from build123d import *

# Parameters (mm, degrees)
SKETCH2_W                                         = 184.171135827
SKETCH2_H                                         = 127
BOSS_EXTRUDE1_DEPTH                               = 4.7625
CSK_FOR_6_FLAT_HEAD_MACHINE_SCREW_100_D           = 4.3053
CSK_FOR_6_FLAT_HEAD_MACHINE_SCREW_100_CSINK_D     = 7.0866
CSK_FOR_6_FLAT_HEAD_MACHINE_SCREW_100_CSINK_ANGLE = 100
CUT_EXTRUDE1_DEPTH                                = 2440.147405433
F_2_CLEARANCE_HOLE1_D                             = 2.7051
CUT_EXTRUDE2_DEPTH                                = 4.7625
FILLET1_R                                         = 25.4
SKETCH10_W                                        = 30.7975
SKETCH10_H                                        = 54.356
CUT_EXTRUDE3_DEPTH                                = 2440.147405433
FILLET2_R                                         = 6.35
CUT_EXTRUDE4_DEPTH                                = 2440.147405433
FILLET3_R                                         = 12.7


with BuildPart() as part:
    # Sketch2 → Boss-Extrude1 (new body)
    with BuildSketch(Plane(origin=(-1e-09, -851.606445574, 6059.494718221), x_dir=(-1, 0, 0), z_dir=(1.0892556339675399e-13, 0.13917310096006327, -0.9902680687415707))):
        with Locations((-199.574242123, -2357.490725166)):
            Rectangle(SKETCH2_W, SKETCH2_H)
    extrude(amount=BOSS_EXTRUDE1_DEPTH)

    # CSK for #6 Flat Head Machine Screw (100)1 (through all)
    with Locations(Plane(origin=(-1e-09, -850.94363368, 6054.778566544), x_dir=(-1, 0, 0), z_dir=(1.0707755897952407e-13, 0.13917310096005847, -0.9902680687415714))):
        with Locations((-115.42617421, -2301.928225166), (-229.72617421, -2301.928225166), (-283.722310037, -2413.053225166)):
            CounterSinkHole(CSK_FOR_6_FLAT_HEAD_MACHINE_SCREW_100_D / 2, CSK_FOR_6_FLAT_HEAD_MACHINE_SCREW_100_CSINK_D / 2, counter_sink_angle=CSK_FOR_6_FLAT_HEAD_MACHINE_SCREW_100_CSINK_ANGLE)

    # Sketch5 → Cut-Extrude1 (cut, through all)
    with BuildSketch(Plane(origin=(-1e-09, -850.94363368, 6054.778566544), x_dir=(-1, 0, 0), z_dir=(1.0707755897952407e-13, 0.13917310096005847, -0.9902680687415714))):
        with BuildLine():
            Line((-195.975000021, -2361.610724808), (-195.975000021, -2336.210724808))
            ThreePointArc((-195.975000021, -2336.210724808), (-183.275000021, -2323.510724808), (-170.575000021, -2336.210724808))
            Line((-170.575000021, -2336.210724808), (-170.575000021, -2361.610724808))
            ThreePointArc((-170.575000021, -2361.610724808), (-183.275000021, -2374.310724808), (-195.975000021, -2361.610724808))
        make_face()
    extrude(amount=-CUT_EXTRUDE1_DEPTH, mode=Mode.SUBTRACT)

    # #2 Clearance Hole1 (through all)
    with Locations(Plane(origin=(-1e-09, -850.94363368, 6054.778566544), x_dir=(-1, 0, 0), z_dir=(1.0707755897952407e-13, 0.13917310096005847, -0.9902680687415714))):
        with Locations((-135.015000021, -2391.392725166), (-160.415000021, -2391.392725166), (-160.415000021, -2330.686725166), (-135.015000021, -2330.686725166), (-204.864100021, -2328.675325166), (-204.864100021, -2403.605325166), (-253.124100021, -2409.955325166), (-253.124100021, -2327.405325166)):
            Hole(F_2_CLEARANCE_HOLE1_D / 2)

    # Sketch9 → Cut-Extrude2 (cut)
    with BuildSketch(Plane(origin=(-1e-09, -850.94363368, 6054.778566544), x_dir=(-1, 0, 0), z_dir=(1.0707755897952407e-13, 0.13917310096005847, -0.9902680687415714))):
        with BuildLine():
            Line((-252.324559302, -2417.852453814), (-282.922769318, -2420.950353814))
            ThreePointArc((-282.922769318, -2420.950353814), (-283.322030383, -2420.980625903), (-283.722310037, -2420.990725166))
            Line((-283.722310037, -2420.990725166), (-107.48867421, -2420.990725166))
            Line((-107.48867421, -2420.990725166), (-107.48867421, -2301.928225166))
            ThreePointArc((-107.48867421, -2301.928225166), (-108.092880421, -2304.96577491), (-109.813514134, -2307.540885241))
            Line((-109.813514134, -2307.540885241), (-127.077500021, -2324.804871128))
            Line((-127.077500021, -2324.804871128), (-127.077500021, -2391.392725166))
            ThreePointArc((-127.077500021, -2391.392725166), (-129.402339945, -2397.005385241), (-135.015000021, -2399.330225166))
            Line((-135.015000021, -2399.330225166), (-159.344404514, -2399.330225166))
            Line((-159.344404514, -2399.330225166), (-202.761165842, -2411.259185244))
            ThreePointArc((-202.761165842, -2411.259185244), (-203.291186027, -2411.385418213), (-203.828617327, -2411.474993637))
            Line((-203.828617327, -2411.474993637), (-252.088617327, -2417.824993637))
            ThreePointArc((-252.088617327, -2417.824993637), (-252.206485588, -2417.839606363), (-252.324559302, -2417.852453814))
        make_face()
        with BuildLine():
            Line((-291.659810037, -2293.990725166), (-291.659810037, -2413.053225166))
            ThreePointArc((-291.659810037, -2413.053225166), (-291.543281919, -2411.69812182), (-291.197118994, -2410.382806226))
            Line((-291.197118994, -2410.382806226), (-260.598908977, -2324.734906226))
            ThreePointArc((-260.598908977, -2324.734906226), (-259.919874258, -2323.303940185), (-258.970238667, -2322.036287154))
            Line((-258.970238667, -2322.036287154), (-235.572312857, -2296.559187154))
            ThreePointArc((-235.572312857, -2296.559187154), (-232.918913397, -2294.661154041), (-229.72617421, -2293.990725166))
            Line((-229.72617421, -2293.990725166), (-291.659810037, -2293.990725166))
        make_face()
        with BuildLine():
            ThreePointArc((-115.42617421, -2293.990725166), (-109.813514134, -2296.31556509), (-107.48867421, -2301.928225166))
            Line((-107.48867421, -2301.928225166), (-107.48867421, -2293.990725166))
            Line((-107.48867421, -2293.990725166), (-115.42617421, -2293.990725166))
        make_face()
        with BuildLine():
            Line((-291.659810037, -2420.990725166), (-283.722310037, -2420.990725166))
            ThreePointArc((-283.722310037, -2420.990725166), (-289.334970113, -2418.665885241), (-291.659810037, -2413.053225166))
            Line((-291.659810037, -2413.053225166), (-291.659810037, -2420.990725166))
        make_face()
    extrude(amount=-CUT_EXTRUDE2_DEPTH, mode=Mode.SUBTRACT)

    # Fillet1
    fillet1_edges = [part.edges().sort_by_distance(p)[0] for p in [
        (127.07750002, -3153.45506956, 5733.586339341),
        (159.344404514, -3227.255147975, 5723.214414719),
    ]]
    fillet(fillet1_edges, radius=FILLET1_R)

    # Sketch10 → Cut-Extrude3 (cut, through all)
    with BuildSketch(Plane(origin=(-1e-09, -850.94363368, 6054.778566544), x_dir=(-1, 0, 0), z_dir=(1.0707755897952407e-13, 0.13917310096005847, -0.9902680687415714))):
        with Locations((-148.826250021, -2361.039725166)):
            Rectangle(SKETCH10_W, SKETCH10_H)
    extrude(amount=-CUT_EXTRUDE3_DEPTH, mode=Mode.SUBTRACT)

    # Fillet2
    fillet2_edges = [part.edges().sort_by_distance(p)[0] for p in [
        (133.42750002, -3162.423782917, 5732.325868879),
        (133.42750002, -3216.250794061, 5724.760975804),
        (164.22500002, -3216.250794061, 5724.760975804),
        (164.22500002, -3162.423782917, 5732.325868879),
    ]]
    fillet(fillet2_edges, radius=FILLET2_R)

    # Sketch11 → Cut-Extrude4 (cut, through all)
    with BuildSketch(Plane(origin=(-1e-09, -850.94363368, 6054.778566544), x_dir=(-1, 0, 0), z_dir=(1.0707755897952407e-13, 0.13917310096005847, -0.9902680687415714))):
        Polygon((-246.774100021, -2333.924628802), (-246.774100021, -2402.715065895), (-211.214100021, -2398.036118527), (-211.214100021, -2334.860418276), align=None)
    extrude(amount=-CUT_EXTRUDE4_DEPTH, mode=Mode.SUBTRACT)

    # Fillet3
    fillet3_edges = [part.edges().sort_by_distance(p)[0] for p in [
        (246.77410002, -3162.486074379, 5732.317114385),
        (211.21410002, -3163.412756814, 5732.186877662),
        (211.21410002, -3225.973635493, 5723.394519553),
        (246.77410002, -3230.607047667, 5722.743335939),
    ]]
    fillet(fillet3_edges, radius=FILLET3_R)


solid = part.part
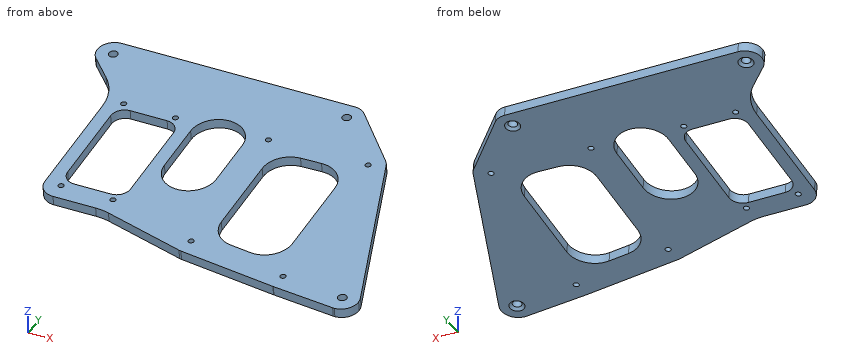
Here's how the part is built. I have some questions about the finished solid (model axes, mm). Coordinates: 2 decimals unless noted, no trailing zeros. Order: outer loops, then holes, each group sorted by start corner. A loop starts at its lowest first (then second) coordinate and runs counter-clockwise, first axis right, second up. Notation, with made-up numbers: (71, 81) -> (89, 81) arc R24 ccw to (89, 108) -> close; hole circle Ø4 at (49.5, -26.5). An arc over 180 degrees is marked (long way). Answer in a Markdown table with one row per item.
(1) I want a section at B-B on x = 216.5. List the corners of the cut face in (y, z) for me, then the cut area to 3 significant figures.
Answer key:
| item | result |
|---|---|
| outline | (-3241.26, 5723.65) -> (-3240.6, 5718.93) -> (-3224.82, 5721.15) -> (-3225.49, 5725.87) -> close; (-3165.78, 5734.26) -> (-3165.12, 5729.54) -> (-3122.61, 5735.52) -> (-3123.27, 5740.23) -> close |
| area | 280 mm^2 |
(2) Please list where these lines run through material, in increasing order: probe 1 along X at (y, z) = (-3191, 5726.75) (1 decimal); probe 2 along X at (y, z) = (-3156, 5732.75); probe 3 along X at (y, z) = (-3223.5, 5722).
Answer key:
| item | result |
|---|---|
| probe 1 | 127.1 to 133.4, 164.2 to 170.6, 195.9 to 211.2, 246.8 to 274.2 |
| probe 2 | 125.82 to 174.09, 192.46 to 204.31, 205.42 to 251.77, 254.48 to 261.57 |
| probe 3 | 128.4 to 214.84, 244.29 to 285.98 |
(3) I want a section at C-C on x = 272.5. List the corners of the cut face in (y, z) for me, then the cut area to 3 significant figures.
Answer key:
| item | result |
|---|---|
| outline | (-3247.95, 5722.71) -> (-3247.29, 5717.99) -> (-3186.04, 5726.6) -> (-3186.71, 5731.32) -> close |
| area | 295 mm^2 |
(4) Will these pins go through, and if not, where does the flat tip stop? pin 1 Ø3 at (y, z) = (-3202, 5728.5) entering from -X; pin 2 Ø5.5 at (y, z) = (-3196.5, 5730) entering from +X; pin 3 Ø8 at (y, z) = (-3193.5, 5728) entering from +X.
Answer key:
| item | result |
|---|---|
| pin 1 | x = 127.08 |
| pin 2 | x = 277.01 |
| pin 3 | x = 276.5 |
(5) I want a section at A-A on x = 173. List the corners of the cut face in (y, z) for me, then the cut area to 3 significant figures.
Answer key:
| item | result |
|---|---|
| outline | (-3231.3, 5725.05) -> (-3230.64, 5720.33) -> (-3196.96, 5725.07) -> (-3197.63, 5729.78) -> close; (-3157.69, 5735.4) -> (-3157.03, 5730.68) -> (-3122.61, 5735.52) -> (-3123.27, 5740.23) -> close |
| area | 327 mm^2 |
